Check sheet for the drawn part. Datum: minimum x, y, z corner. Units: mm. A direction names the side the tool comes from. Give positions to 0.01 mm unless a question says otherwise; leave off trailing zeros. Loops run counter-clockwise (first coordinate to the right, second up) from the corner with the lowest first, then second, coordinate; pieces in that order, holes last. Notation, with made-up numbers: (-38.75, 41.5) -> (-32.75, 41.5) arc R9 cw to (-32.75, 50.5) -> close; hole circle Ø6 at (28, 33). An arc over 180 degrees is marked (long way). One line per question, with ' | ' between items.
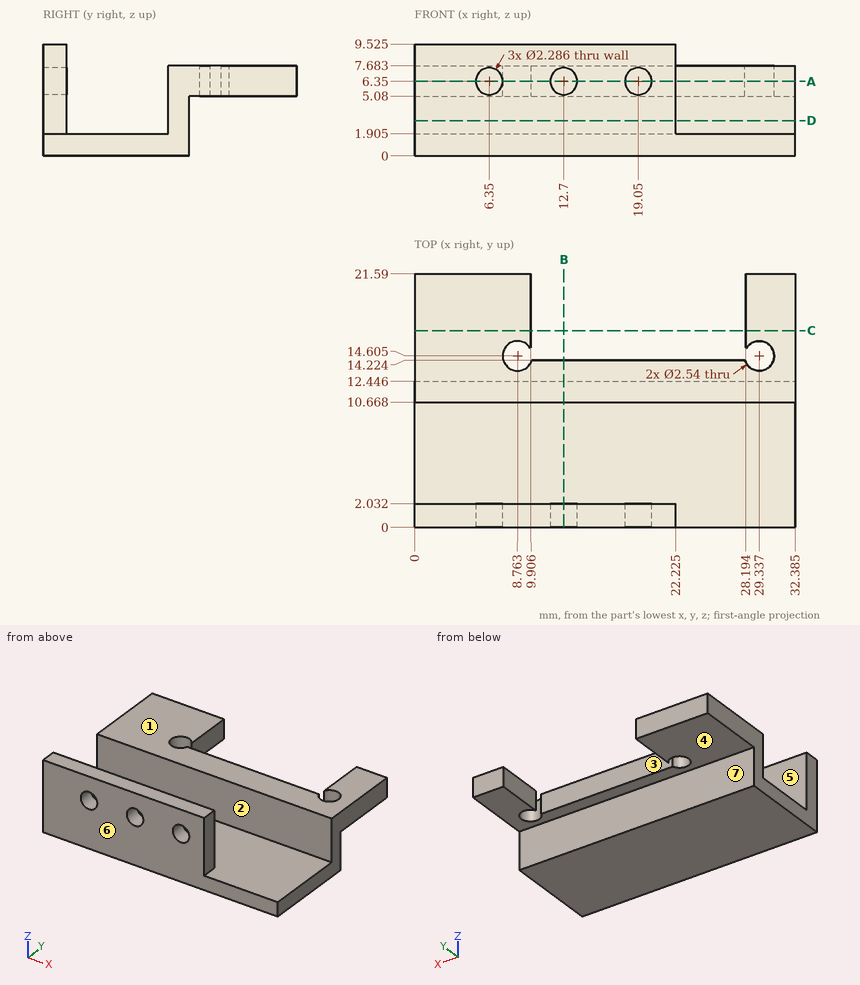
Item 1: Scan lines: probe 1 along Y at (x, z) = (8, 6); probe 2 along Y at (x, z) = (12.5, 3.5) (1 decimal); probe 3 along Z at (x, y) = (6.35, 1.25) (1 decimal). Record each from-to range of solid material in increasing order.
Result:
probe 1: 0 to 2.03, 10.67 to 13.59, 15.62 to 21.59 | probe 2: 0 to 2, 10.7 to 12.4 | probe 3: 0 to 5.2, 7.5 to 9.5
Item 2: Depth check by flat-ended pin: pin 1 Ø4.5 at (x, y) = (16.5, 16) entering from -Z; pin 2 Ø1 at (y, z) = (1.5, 6) entering from +X (1 decimal); pin 3 Ø0.8 at (x, z) = (19, 7) entering from +Y; pin 4 Ø4 at (x, y) = (7, 13) entering from -Z. Enter the tip coordinate at first touch or a pass-through.
Result:
pin 1: z = 5.08 | pin 2: x = 22.2 | pin 3: y = 14.22 | pin 4: z = 0
Item 3: Set-up check for the marked faces 1, 2, 3 and 4: record each of +Z, -Z, +X, -X, +Y, -Y from which the full face is reachable in a straight line by a thin tool's end or side.
Result:
face 1: +Z, +X, -X, +Y | face 2: +Z, +X, -X | face 3: +Z, -Z, +Y | face 4: -Z, +X, -X, +Y
Item 4: Sectioned sample at A-A (z = 6.35). Record the cut outline in (x, y) (1 decimal), plus the area to 3 significant figures.
Result:
outline: (0, 0) -> (5.2, 0) -> (5.2, 2) -> (0, 2) -> close; (0, 10.7) -> (32.4, 10.7) -> (32.4, 21.6) -> (28.2, 21.6) -> (28.2, 15.2) arc R1.3 cw (long way) to (28.1, 14.2) -> (10, 14.2) arc R1.3 cw (long way) to (9.9, 15.2) -> (9.9, 21.6) -> (0, 21.6) -> close; (7.5, 0) -> (11.6, 0) -> (11.6, 2) -> (7.5, 2) -> close; (13.8, 0) -> (17.9, 0) -> (17.9, 2) -> (13.8, 2) -> close; (20.2, 0) -> (22.2, 0) -> (22.2, 2) -> (20.2, 2) -> close | area: 240 mm2
Item 5: Release check for a two-part mould opening along Y. For the marked faces 5, 6 and 7 record: pulls with the +Y half, pulls with the -Y half, needs draft (parallel to the pull), parting line crosses it, or undercut.
Result:
face 5: undercut | face 6: pulls with the -Y half | face 7: pulls with the +Y half
Item 6: Sectioned sample at B-B (x = 12.7). Record the cut outline in (y, z) (1 decimal).
Result:
outline: (0, 0) -> (12.4, 0) -> (12.4, 5.1) -> (14.2, 5.1) -> (14.2, 7.7) -> (10.7, 7.7) -> (10.7, 1.9) -> (2, 1.9) -> (2, 5.2) -> (0, 5.2) -> close; (0, 7.5) -> (2, 7.5) -> (2, 9.5) -> (0, 9.5) -> close
Item 7: Sectioned sample at D-D (z = 3). Record the cut outline in (x, y) (1 decimal).
Result:
outline: (0, 0) -> (22.2, 0) -> (22.2, 2) -> (0, 2) -> close; (0, 10.7) -> (32.4, 10.7) -> (32.4, 12.4) -> (0, 12.4) -> close
Item 8: Sectioned sample at C-C (y = 16.75). Record the cut outline in (x, z) (1 decimal), plus the area to 3 significant figures.
Result:
outline: (0, 5.1) -> (9.9, 5.1) -> (9.9, 7.7) -> (0, 7.7) -> close; (28.2, 5.1) -> (32.4, 5.1) -> (32.4, 7.7) -> (28.2, 7.7) -> close | area: 36.7 mm2
